```python
from build123d import *

# Parameters (mm, degrees)
SKETCH1_R           = 14
SKETCH1_R_2         = 8
BOSS_EXTRUDE1_DEPTH = 10
SKETCH1_3_R         = 14
SKETCH1_3_R_2       = 8
BOSS_EXTRUDE2_DEPTH = 32.5
SKETCH2_R           = 2.5
CUT_EXTRUDE1_DEPTH  = 32.5


with BuildPart() as part:
    # Sketch1 → Boss-Extrude1 (new body)
    with BuildSketch(Plane(origin=(0, 0, 0), x_dir=(1, 0, 0), z_dir=(0, 1, 0))):
        with BuildLine():
            ThreePointArc((20, 13.446560899), (0, 24.1), (-20, 13.446560899))
            Line((-20, 13.446560899), (-20, -13.446560899))
            ThreePointArc((-20, -13.446560899), (0, -24.1), (20, -13.446560899))
            Line((20, -13.446560899), (20, 13.446560899))
        make_face()
        Circle(SKETCH1_R, mode=Mode.SUBTRACT)
        Circle(SKETCH1_R)
        Circle(SKETCH1_R_2, mode=Mode.SUBTRACT)
    extrude(amount=BOSS_EXTRUDE1_DEPTH)

    # Sketch1_3 → Boss-Extrude2 (add)
    with BuildSketch(Plane(origin=(0, 0, 0), x_dir=(1, 0, 0), z_dir=(0, 1, 0))):
        Circle(SKETCH1_3_R)
        Circle(SKETCH1_3_R_2, mode=Mode.SUBTRACT)
    extrude(amount=-BOSS_EXTRUDE2_DEPTH)

    # Sketch2 → Cut-Extrude1 (cut)
    with BuildSketch(Plane(origin=(0, 10, 0), x_dir=(1, 0, 0), z_dir=(0, 1, 0))):
        with Locations((0, -18.75)):
            Circle(SKETCH2_R)
        with Locations((-13.258252147, -13.258252147)):
            Circle(SKETCH2_R)
        with Locations((-13.258252147, 13.258252147)):
            Circle(SKETCH2_R)
        with Locations((0, 18.75)):
            Circle(SKETCH2_R)
        with Locations((13.258252147, 13.258252147)):
            Circle(SKETCH2_R)
        with Locations((13.258252147, -13.258252147)):
            Circle(SKETCH2_R)
    extrude(amount=-CUT_EXTRUDE1_DEPTH, mode=Mode.SUBTRACT)


solid = part.part
```
Here's how the part is built. I have some questions about the finished solid (model axes, mm). A direction names the side the tool comes from. Give positions to 0.01 mm unless a question says otherwise; leave off trailing zeros. Order: outer loops, then holes, each group sorted by start corner. A loop starts at its lowest first (then second) coordinate and runs counter-clockwise, first axis right, second up. Notation, with made-up numbers: M 7,-7.5 L 32,-7.5 A17 ccw 32,7.5 Z; hole C 51.5,41.5 d3. An arc over 180 degrees is marked long. Use a Markdown table: item, result. Add a question column.
1. Suppose I cut it at A-A (x = 0). List the corners of the cut face in (y, z) for me, and give its area (3 significant figures).
2. For pin 1 Ø1.5 at (y, z) = (2, 17) entering from -X; pin 2 Ø5 at (x, y) = (6.5, -12.5) entering from -Z; pin 3 Ø6.5 at (x, z) = (0, -18.75) entering from +Y; pin 4 Ø3 at (y, z) = (-6, -0.5) entering from +X, each with a flat end and sliding along its axis, tell me the tip position at first contact or that it passes through.
3. On a 3-axis mill with a long thin cutter (end or side, diameter ignored), from which of +Z, -Z, +X, -X, +Y, -Y can I reach the whole of each face in a straight line? I mean faces 4 (the flat face through (9, 0, -11)), 5 (the cylindrical face through (-0.33, 5.07, -21.23)). Say none if no direction works.
4. Suppose I cut it at C-C (y = 7). List the corners of the cut face in (x, z) for me, and give its area (3 significant figures).
5. Suppose I cut it at D-D (x = -5.5). List the corners of the cut face in (y, z) for me.
6. Suppose I cut it at B-B (z = 0). List the corners of the cut face in (x, y) for me.
7. I need wall thicknesses on probe 1 along X at (y, z) = (-13, 0); probe 2 along X at (y, z) = (8.5, 0). Which ranges of each line are inside material? Lowest first, please. Write a range as from..to.
8. If we mould it in two halves opening along Z, with no side actions, what happens to faces 1 (the cylindrical face through (-15.756, 5.07, 13.148)), 2 (the flat face through (9, 10, 0)), 3 (the cylindrical face through (12.932, -16.022, 5.362))? For each: +Z half, -Z half, draft (parallel to the pull), parting line (faces both ways), or undercut.
Results list:
| question | item | result |
|---|---|---|
| 1 | outline | M -32.5,-14 L 0,-14 L 0,-16.25 L 10,-16.25 L 10,-8 L -32.5,-8 Z; M -32.5,8 L 10,8 L 10,16.25 L 0,16.25 L 0,14 L -32.5,14 Z; M 0,-24.1 L 10,-24.1 L 10,-21.25 L 0,-21.25 Z; M 0,21.25 L 10,21.25 L 10,24.1 L 0,24.1 Z |
| 1 | area | 612 mm² |
| 2 | pin 1 | stops at x = -17.8 |
| 2 | pin 2 | stops at z = -13.42 |
| 2 | pin 3 | stops at y = 10 |
| 2 | pin 4 | stops at x = 14 |
| 3 | face 4 | -Y |
| 3 | face 5 | +Y, -Y |
| 4 | outline | M -20,-13.45 A24.1 ccw 20,-13.45 L 20,13.45 A24.1 ccw -20,13.45 Z; hole C -13.26,-13.26 d5; hole C -13.26,13.26 d5; hole C 0,0 d16; hole C 0,-18.75 d5; hole C 0,18.75 d5; hole C 13.26,-13.26 d5; hole C 13.26,13.26 d5 |
| 4 | area | 1,360 mm² |
| 5 | outline | M -32.5,-12.87 L 0,-12.87 L 0,-23.46 L 10,-23.46 L 10,-5.81 L -32.5,-5.81 Z; M -32.5,5.81 L 10,5.81 L 10,23.46 L 0,23.46 L 0,12.87 L -32.5,12.87 Z |
| 6 | outline | M -20,0 L -14,0 L -14,-32.5 L -8,-32.5 L -8,10 L -20,10 Z; M 8,-32.5 L 14,-32.5 L 14,0 L 20,0 L 20,10 L 8,10 Z |
| 7 | probe 1 | x = -14..-8, 8..14 |
| 7 | probe 2 | x = -20..-8, 8..20 |
| 8 | face 1 | undercut |
| 8 | face 2 | draft |
| 8 | face 3 | parting line |
